For this review, take the finished solid that the model builds, in its own axes (mm). A direction names the side the tool comes from. Give positions to 0.01 mm unless a question says otherwise; leave off trailing zeros. Write each loop counter-clockwise with the first axis right and the second up, starting at its lowest first coordinate (ties: lowest second). Pieces come first, ordered by that corner, then holes.
Q1. Insertion check: P1, Ø4, axis at x = -1.5, y = 0, coming from the +Z side; P2, Ø1.5, axis at x = 0, z = 2.5, coming from the -Y side. Each pin has a flat end and moves straight along its axis. Give the tip position at first contact, or say it passes through.
Q2. We need section D-D (x = -2.75). Write out the cut boundary in (y, z).
Q3. We need section A-A (x = 0). Write out the cut boundary in (y, z), then the cut area to 3 significant figures.
Q4. We need section C-C (z = 1.3). Write out the cut boundary in (x, y), then the cut area to 3 significant figures.
Q5. For line 1 (X direction, y = -2.5, z = 1.2); line 2 (Y direction, x = 0.5, z = 1.15); line 3 (X direction, y = 1.75, z = 1.05), list the stretches that pass through material, from the lowest coordinate up.
Q6. Mouldability with a two-part tool opening along X and no side actions: class faces 1 (the flat face through (2.1, -2, 1)), 2 (the flat face through (1, 2, 2)), 3 (the flat face through (4, 7, 1)) as released by +X, released by -X, zero draft, split by the parting line, or undercut.
Q7. Machinability: for faces 4 (the flat face through (0, 15.6, 2)), 5 (the cylindrical face through (0, 18, 2)), 6 (the flat face through (-2.1, -2, 1)), which of the approach directions +Z, -Z, +X, -X, +Y, -Y give a long, thin tool a straight path to every point of the face, cutting with its end or side? Answer none if there is none.
Q8. We need section B-B (y = 1.25). Write out the cut boundary in (x, z), then the cut area to 3 significant figures.
```python
from build123d import *

# Parameters (mm, degrees)
BOSS_EXTRUDE1_DEPTH = 3.6
CHAMFER1_SIZE       = 1.131371061
CHAMFER1_SIZE2      = 1.131370771
BOSS_EXTRUDE2_DEPTH = 2


with BuildPart() as part:
    # Sketch1 → Boss-Extrude1 (new body)
    with BuildSketch(Plane(origin=(0, 0, 0), x_dir=(-1, 0, 0), z_dir=(0, 0, -1))):
        with BuildLine():
            Line((-4, 14), (-4, 4.000000018))
            Line((-4, 4.000000018), (4, 4.000000018))
            Line((4, 4.000000018), (4, 14))
            ThreePointArc((4, 14), (0, 18), (-4, 14))
        make_face()
        Polygon((-0.92376, 12.400000746), (-1.84752, 14), (-0.92376, 15.599999254), (0.92376, 15.599999254), (1.84752, 14), (0.92376, 12.400000746), align=None, mode=Mode.SUBTRACT)
    extrude(amount=-BOSS_EXTRUDE1_DEPTH)

    # Chamfer1
    chamfer1_edges = [part.edges().sort_by_distance(p)[0] for p in [
        (0, 4.000000018, 3.6),
    ]]
    chamfer1_side = [part.faces().sort_by_distance(p)[0] for p in [
        (0, 4.000000018, 1.8),
    ]]
    chamfer(chamfer1_edges, length=CHAMFER1_SIZE, length2=CHAMFER1_SIZE2, reference=chamfer1_side[0])

    # Sketch6 → Boss-Extrude2 (add)
    with BuildSketch(Plane(origin=(0, 0, 0), x_dir=(-1, 0, 0), z_dir=(0, 0, -1))):
        with BuildLine():
            Line((-4, -4), (-2.1, -4))
            Line((-2.1, -4), (-2.1, -0.156392755))
            ThreePointArc((-2.1, -0.156392755), (0, 1.943607245), (2.1, -0.156392755))
            Line((2.1, -0.156392755), (2.1, -4))
            Line((2.1, -4), (4, -4))
            Line((4, -4), (4, 4.000000018))
            Line((4, 4.000000018), (-4, 4.000000018))
            Line((-4, 4.000000018), (-4, -4))
        make_face()
    extrude(amount=-BOSS_EXTRUDE2_DEPTH)


solid = part.part
```
Computed:
1. P1: stops at z = 2
1. P2: stops at y = 1.87
2. outline: (-4, 0) - (16.9, 0) - (16.9, 3.6) - (5.13, 3.6) - (4, 2.47) - (4, 2) - (-4, 2) - close
3. outline: (1.94, 0) - (12.4, 0) - (12.4, 3.6) - (5.13, 3.6) - (4, 2.47) - (4, 2) - (1.94, 2) - close; (15.6, 0) - (18, 0) - (18, 3.6) - (15.6, 3.6) - close
3. area: 42.4 mm2
4. outline: (-4, -4) - (-2.1, -4) - (-2.1, -0.16) arc R2.1 cw to (2.1, -0.16) - (2.1, -4) - (4, -4) - (4, 14) arc R4 ccw to (-4, 14) - close; hole (-1.85, 14) - (-0.92, 12.4) - (0.92, 12.4) - (1.85, 14) - (0.92, 15.6) - (-0.92, 15.6) - close
4. area: 137 mm2
5. line 1: x = -4 to -2.1, 2.1 to 4
5. line 2: y = 1.88 to 12.4, 15.6 to 17.97
5. line 3: x = -4 to -0.88, 0.88 to 4
6. face 1: undercut
6. face 2: zero draft
6. face 3: released by +X
7. face 4: +Z, -Z
7. face 5: +Z, -Z, +Y
7. face 6: +Z, -Z, -Y
8. outline: (-4, 0) - (-1.56, 0) - (-1.56, 2) - (-4, 2) - close; (1.56, 0) - (4, 0) - (4, 2) - (1.56, 2) - close
8. area: 9.76 mm2
